Autodesk Fusion 360 part; units mm, degrees
sketch "Sketch1" plane through (0, 0, 0) normal (0, 1, 0) x (1, 0, 0)
  line L0 (-36, 0) -> (40, 0) construction
  arc A0 (-32, 0) -> (0, -32) centre (0, 0) ccw
  arc A1 (-22, 0) -> (0, -22) centre (0, 0) ccw
  line L1 (0, -32) -> (0, -22)
  line L2 (-22, 0) -> (-32, 0)
  dimension "d3" = 22
  dimension "d4" = 32
revolve "Revolve1" add sketch "Sketch1" angle 360 about axis through (0, 0, 1.75) along (0, 0, 1)
sketch "Sketch2" plane through (0, 0, 0) normal (0, 0, -1) x (1, 0, 0)
  circle A0 centre (0, 0) radius 32
  circle A1 centre (0, 0) radius 22
  circle A2 centre (0, 0) radius 25.1968
  circle A3 centre (0, 0) radius 28.956
  dimension "d6" = 50.3936
  dimension "d7" = 57.912
extrude "Extrude1" cut sketch "Sketch2" against normal blind 2.921 contours A3
sketch "Sketch3" plane through (0, 0, 0) normal (0, 0, -1) x (1, 0, 0)
  circle A0 centre (0, 0) radius 32
  circle A1 centre (0, 0) radius 28.956
  circle A2 centre (0, 0) radius 37
  dimension "d10" = 74
extrude "Extrude2" add sketch "Sketch3" against normal blind 5 contours A0 | A2
fillet "Fillet1" radius 0.05 2 edges at (-23.4917, 9.1116, 0) (-26.9965, -10.4709, 0)
Input: part model. Units: mm. Frame: model coordinates. A direction names the side the tool comes from. Coordinates: 2 decimals unless noted, no trailing zeros. Write each loop counter-clockwise with the first axis right and the second up, starting at its lowest first coordinate (ties: lowest second). Pieces come first, ordered by that corner, then holes. Notation, with made-up numbers: (82, 75.5) -> (89, 75.5) arc R31 cw to (89, 104.5) -> close; hole circle Ø8 at (-36, 5). An arc over 180 degrees is marked (long way). Answer as a JSON object with one key per item and string values.
1. Section D-D on z = 24. Return the cut outline in (x, y), then the cut area to 3 significant figures.
Result set:
{"outline": "circle Ø42.33 at (0, 0)", "area": "1,410 mm2"}
2. Mould query, pull axis Y, two halves, no side actions, for faces 1 (the face through (-16.3, 24.5, 0)), 2 (the face through (-3.77, -28.71, 1.47)), 3 (the face through (-8.02, 36.12, 2.46)). Classes: released by +Y, released by -Y, zero draft, split by the parting line, or undercut.
Result set:
{"face 1": "zero draft", "face 2": "undercut", "face 3": "split by the parting line"}
3. Section C-C on z = 4. Return the cut outline in (x, y).
Result set:
{"outline": "circle Ø74 at (0, 0); hole circle Ø43.27 at (0, 0)"}
4. Section A-A on y = 0. Return the cut outline in (x, z), then the cut area to 3 significant figures.
Result set:
{"outline": "(-37, 0) -> (-29.01, 0) arc R0.05 ccw to (-28.96, 0.05) -> (-28.96, 2.92) -> (-25.2, 2.92) -> (-25.2, 0.05) arc R0.05 ccw to (-25.15, 0) -> (-22, 0) arc R22 cw to (22, 0) -> (25.15, 0) arc R0.05 ccw to (25.2, 0.05) -> (25.2, 2.92) -> (28.96, 2.92) -> (28.96, 0.05) arc R0.05 ccw to (29.01, 0) -> (37, 0) -> (37, 5) -> (31.61, 5) arc R32 ccw to (-31.61, 5) -> (-37, 5) -> close", "area": "878 mm2"}
5. Access query for faces 4 (the face through (27, -17, 5)), 5 (the face through (-19.995, 15.332, 1.465)), 6 (the face through (0.1, 22.2, 0)). Directions: +Z, -Z, +X, -X, +Y, -Y. A direction counts if a zero-diameter tool reaches every point of the face in a straight line with its end or side. Return the directions, or none.
Result set:
{"face 4": "+Z", "face 5": "-Z", "face 6": "-Z, +X, -X, +Y, -Y"}
6. Material intervals for line 1 (Y direction, x = 0, z = 0.95); line 2 (X direction, y = -7, z = 2.5); line 3 (X direction, y = 0, z = 1.45), sorted ascending. Write a range as from..to.
Result set:
{"line 1": "y = -37..-28.96, -25.2..-21.98, 21.98..25.2, 28.96..37", "line 2": "x = -36.33..-28.1, -24.2..-20.71, 20.71..24.2, 28.1..36.33", "line 3": "x = -37..-28.96, -25.2..-21.95, 21.95..25.2, 28.96..37"}
7. First-contact query: P1, Ø1.5, axis at x = -7.5, z = 19, coming from the -Y side; P2, Ø4, axis at x = -27, y = 25.5, coming from the +Z side; P3, Ø12, axis at x = 3.5, z = 27, coming from the -Y side. Flat tips, straight axial feed; report the tip coordinate or a pass-through.
Result set:
{"P1": "stops at y = -25.24", "P2": "stops at z = 5", "P3": "stops at y = -23.95"}
